Part model, mm, in its own coordinate system. Face numbers are marked on the shaded views. Give positions to 0.01 mm unless a question says otherwise; leave off trailing zeros. Order: outer loops, then holes, each group sorted by start corner. A loop starts at its lowest first (then second) coordinate and runs counter-clockwise, first axis right, second up. Notation, with made-up numbers: (88, -25) - (122, -25) arc R15 ccw to (122, -13) - close; hole circle Ø7 at (74, 48). An arc over 180 degrees is marked (long way). One line per item, written item: value.
```python
from build123d import *

# Parameters (mm, degrees)
F0_W     = 100
F0_H     = 100
F1_DEPTH = 4
F2_R     = 0.5
F3_R     = 2.45
F4_DEPTH = 20
F5_R     = 4.5
F5_R_2   = 13.5
F5_R_3   = 2
F5_R_4   = 5.5
F5_R_5   = 18
F5_R_6   = 15.5
F5_R_7   = 8.5
F6_DEPTH = 25


with BuildPart() as f1:
    # F0 (on Top) → F1 (new body)
    with BuildSketch(Plane.XY):
        with Locations((-18.745929, -1.397985)):
            Rectangle(F0_W, F0_H)
    extrude(amount=F1_DEPTH)

    # F2
    f2_edges = [f1.edges().sort_by_distance(p)[0] for p in [
        (-68.745929, 48.602015, 2),
        (31.254071, 48.602015, 2),
        (31.254071, -51.397985, 2),
        (-68.745929, -51.397985, 2),
    ]]
    fillet(f2_edges, radius=F2_R)

    # F3 (on face) → F4 (join)
    with BuildSketch(Plane.XY.offset(4)):
        with Locations((-63.745929, 43.602015)):
            Circle(F3_R)
        with Locations((26.254071, 43.602015)):
            Circle(F3_R)
        with Locations((-63.745929, -46.397985)):
            Circle(F3_R)
        with Locations((26.254071, -46.397985)):
            Circle(F3_R)
    extrude(amount=F4_DEPTH)

    # F5 (on face) → F6 (cut)
    with BuildSketch(Plane.XY.offset(4)):
        with Locations((-51.634617, 39.038464)):
            Circle(F5_R)
        with Locations((-26.057692, 32.602015)):
            Circle(F5_R_2)
        with Locations((0, 39.038464)):
            Circle(F5_R_3)
        with Locations((8.75, 39.038464)):
            Circle(F5_R_3)
        with Locations((17.78846, 39.038464)):
            Circle(F5_R_3)
        with Locations((21.057691, 19.423077)):
            Circle(F5_R_4)
        with Locations((-4.745929, 4.602015)):
            Circle(F5_R_5)
        with Locations((-44.745929, 4.602015)):
            Circle(F5_R_5)
        with Locations((-41.826926, -32.397985)):
            Circle(F5_R_6)
        with Locations((-6.826926, -32.397985)):
            Circle(F5_R_6)
        with Locations((20.673078, -13.653847)):
            Circle(F5_R_7)
        with Locations((20.673078, -32.397985)):
            Circle(F5_R_7)
    extrude(amount=-F6_DEPTH, mode=Mode.SUBTRACT)


solid = f1.part
```
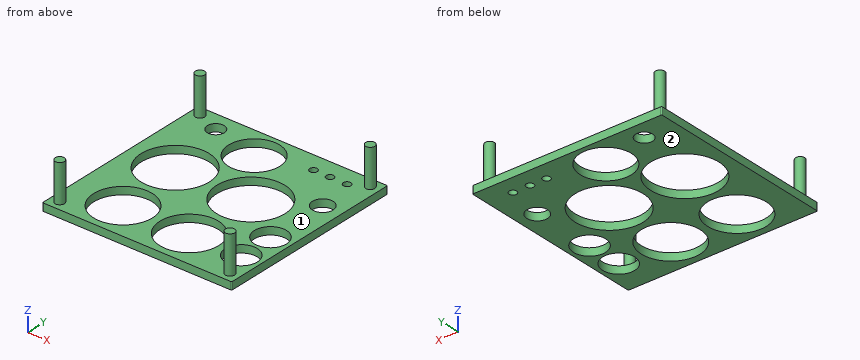
1) Slice it at B-B on y = -29. Write the cut outline in (x, z), then the cut area to 3 significant figures.
Answer:
outline: (-68.75, 0) - (-56.95, 0) - (-56.95, 4) - (-68.75, 4) - close; (-26.7, 0) - (-21.95, 0) - (-21.95, 4) - (-26.7, 4) - close; (8.3, 0) - (12.88, 0) - (12.88, 4) - (8.3, 4) - close; (28.46, 0) - (31.25, 0) - (31.25, 4) - (28.46, 4) - close
area: 95.7 mm2
2) Two-plate mould, pull along Y, no slides. Class the marked faces 1 and 2: pulls with the +Y half, pulls with the -Y half, needs draft (parallel to the pull), parting line crosses it, or undercut.
Answer:
face 1: undercut
face 2: needs draft
3) Slice it at C-C on z = 2. Count the separate pieces of the cut face and the enclosed holes in it, then the cut area to 3 significant figures.
Answer:
separate pieces: 1
enclosed holes: 12
area: 5,230 mm2
4) Slice it at A-A on x = 0. Write the cut outline in (y, z), then the cut area to 3 significant figures.
Answer:
outline: (-51.4, 0) - (-46.31, 0) - (-46.31, 4) - (-51.4, 4) - close; (-18.48, 0) - (-12.76, 0) - (-12.76, 4) - (-18.48, 4) - close; (21.97, 0) - (37.04, 0) - (37.04, 4) - (21.97, 4) - close; (41.04, 0) - (48.6, 0) - (48.6, 4) - (41.04, 4) - close
area: 134 mm2
5) Wall check: line 1 along Y through (x, z) = (8.75, 2.6); line 2 along Z through (x, y) = (-12, 30.5); line 3 along X through (y, z) = (-47, 19.75). Give the ranges that are in metal, low to high. Write a range as [from, to].
Answer:
line 1: y = [-51.4, -7.31], [16.51, 37.04], [41.04, 48.6]
line 2: z = [0, 4]
line 3: x = [-66.12, -61.37], [23.88, 28.63]
6) Slice it at D-D on z = 7.25. Write the cut outline in (x, y).
Answer:
outline: circle Ø4.9 at (-63.75, -46.4); circle Ø4.9 at (-63.75, 43.6); circle Ø4.9 at (26.25, -46.4); circle Ø4.9 at (26.25, 43.6)
7) Drop a flat-ended pin along its axis: P1, Ø11.5, axis at x = -51.63, y = 39.04, coming from the +Z side. Give the stop position or say it passes through.
Answer:
P1: stops at z = 4
